from build123d import *

# Parameters (mm, degrees)
F2_DEPTH  = 10
F3_W      = 29.145509
F3_H      = 20.968225
F4_DEPTH  = 25.4
F5_R      = 50.931249
F6_DEPTH  = 25.4
F6_FACE_R = 50.931249
F7_DEPTH  = 25


with BuildPart() as f2:
    # F0 (on Right) → F2 (new body)
    with BuildSketch(Plane.YZ):
        Polygon((-16.064236, 31.052269), (-16.064236, 32.037951), (32.617681, 32.037951), (32.617681, 35.078097), (-63.268401, 35.078097), (-63.268401, -20.898964), (32.617681, -20.898964), (32.617681, 31.052269), align=None)
    extrude(amount=-F2_DEPTH)

    # F3 (on face) → F4 (cut)
    with BuildSketch(Plane(origin=(-10, 0, 0), x_dir=(0, -1, 0), z_dir=(-1, 0, 0))):
        with Locations((-5.355574, 10.484113)):
            Rectangle(F3_W, F3_H)
    extrude(amount=-F4_DEPTH, mode=Mode.SUBTRACT)

    # F5 (on Right) → F6 (join)
    with BuildSketch(Plane.YZ):
        with Locations((54.566488, 39.468978)):
            Circle(F5_R)
    extrude(amount=F6_DEPTH)

    # F6_face (on face) → F7 (join)
    with BuildSketch(Plane(origin=(25.4, 54.566488, 39.468978), x_dir=(0, 1, 0), z_dir=(1, 0, 0))):
        Circle(F6_FACE_R)
    extrude(amount=-F7_DEPTH)


solid = f2.part
Input: part model. Units: mm. Frame: model coordinates. A direction names the side the tool comes from. Round coordinates to 2 decimals unless told otherwise and drop trailing zeros. Loops run counter-clockwise (first coordinate to the right, second up) from the corner with the lowest first, then second, coordinate; pieces in that order, holes last. Notation, with made-up numbers: (65.5, -33.5) -> (109.5, -33.5) arc R17 ccw to (109.5, -0.5) -> close; hole circle Ø4 at (54.5, 13). An arc over 180 degrees is marked (long way). Answer as a JSON object with one key per item and string values. Group by question number.
1) Ray query, L1, parallel to Z at x = -5, y = -7; L2, parallel to X at y = 52, z = -2; L3, parallel to X at y = -1, z = 34.5. Return the intervals inside material, ascending.
2) Section query D-D on y = 28. Output: boundary loops of the cut face in (x, z).
3) Section query C-C on z = 10. Output: boundary loops of the cut face in (x, y), plus the area to 3 significant figures.
4) Section query B-B on x = -3.5. Output: boundary loops of the cut face in (y, z).
5) Pin query (flat end, axial travel): pin 1 (10 mm diameter, centred on x = 15.5, z = 3.5, fed in from -Y); pin 2 (3 mm diameter, centred on x = -4.5, y = 10, fed in from +Z); pin 3 (10 mm diameter, centred on x = -2.5, y = 27.5, fed in from +Z). Return the tip coordinate at first contact, or that it passes through.
6) Section query A-A on y = -6. Output: boundary loops of the cut face in (x, z), plus the area to 3 significant figures.
7) Reachability of faces 1 (the flat face through (0, 15, 14)), 2 (the flat face through (-5, -15, 35.078)), 3 (the flat face through (-5, 32.618, 5)) from +Z, -Z, +X, -X, +Y, -Y: full face, straight path, thin tool, end or side. Return the list, or none.
8) Draft query along Y for faces 4 (the flat face through (-5, 6, 0)), 5 (the cylindrical face through (12.52, 14.15, 8.48)), 6 (the flat face through (-5, 8, 32.038)). Return one class per face: +Y half, -Y half, draft (parallel to the pull), parting line (faces both ways), or undercut.
Reply:
{
 "1": {"L1": "z = -20.9 to 0, 20.97 to 31.05, 32.04 to 35.08", "L2": "x = 0 to 25.4", "L3": "x = -10 to 0"},
 "2": {"outline": "(-10, -20.9) -> (0, -20.9) -> (0, -3.98) -> (25.4, -3.98) -> (25.4, 82.92) -> (0, 82.92) -> (0, 35.08) -> (-10, 35.08) -> (-10, 32.04) -> (0, 32.04) -> (0, 31.05) -> (-10, 31.05) -> close"},
 "3": {"outline": "(-10, -63.27) -> (0, -63.27) -> (0, -9.22) -> (-10, -9.22) -> close; (-10, 19.93) -> (0, 19.93) -> (0, 13.03) -> (25.4, 13.03) -> (25.4, 96.11) -> (0, 96.11) -> (0, 32.62) -> (-10, 32.62) -> close", "area": "2,780 mm2"},
 "4": {"outline": "(-63.27, -20.9) -> (32.62, -20.9) -> (32.62, 31.05) -> (-16.06, 31.05) -> (-16.06, 32.04) -> (32.62, 32.04) -> (32.62, 35.08) -> (-63.27, 35.08) -> close; hole (-9.22, 0) -> (19.93, 0) -> (19.93, 20.97) -> (-9.22, 20.97) -> close"},
 "5": {"pin 1": "stops at y = 14.13", "pin 2": "stops at z = 35.08", "pin 3": "stops at z = 85.04"},
 "6": {"outline": "(-10, -20.9) -> (0, -20.9) -> (0, 0) -> (-10, 0) -> close; (-10, 20.97) -> (0, 20.97) -> (0, 31.05) -> (-10, 31.05) -> close; (-10, 32.04) -> (0, 32.04) -> (0, 35.08) -> (-10, 35.08) -> close", "area": "340 mm2"},
 "7": {"face 1": "-X", "face 2": "+Z, -X, +Y, -Y", "face 3": "+Z, -Z, -X, +Y"},
 "8": {"face 4": "undercut", "face 5": "parting line", "face 6": "draft"}
}
